```python
from build123d import *
from OCP.BRepFilletAPI import BRepFilletAPI_MakeChamfer

# Parameters (mm, degrees)
SKETCH1_W                 = 5
SKETCH1_H                 = 1.629773482
SKETCH1_H_2               = 1.605700765
BOSS_EXTRUDE21_DEPTH      = 1.5
BOSS_EXTRUDE22_DEPTH      = 0.0001
BOSS_EXTRUDE22_DEPTH_BACK = 5
SKETCH4_W                 = 13.038345926
SKETCH4_H                 = 1.27322458
SKETCH5_W                 = 13.038345926
SKETCH5_H                 = 1.75
BOSS_EXTRUDE23_DEPTH      = 1.5
SKETCH6_W                 = 3.309716912
SKETCH6_H                 = 6.42211522
SKETCH6_W_2               = 3.309716913
BOSS_EXTRUDE24_DEPTH      = 3
SKETCH8_W                 = 3.309716912
SKETCH8_H                 = 1.8
SKETCH8_W_2               = 3.309716913
BOSS_EXTRUDE26_DEPTH      = 1.5
FILLET1_R                 = 1
FILLET2_R                 = 1
CHAMFER1_SIZE             = 3
CHAMFER1_SIZE_2           = 5.412143266


with BuildPart() as part:
    # Sketch1 → Boss-Extrude21 (new body)
    # profile 1 of 3: a face of its own
    with BuildSketch(Plane(origin=(0, 0, 0), x_dir=(1, 0, 0), z_dir=(0, 1, 0))):
        with Locations((9.977336143, 2.209185976)):
            Rectangle(SKETCH1_W, SKETCH1_H)
    # profile 2 of 3: a face of its own
    with BuildSketch(Plane(origin=(0, 0, 0), x_dir=(1, 0, 0), z_dir=(0, 1, 0))):
        Polygon((-7.422672964, -10.702702703), (-20.313450574, -10.702702703), (-20.313450574, -9.652730884), (13.867336143, -9.652730884), (13.867336143, -10.702702703), (0.977336143, -10.702702703), (0.977336143, -11.975927283), (21.477336143, -11.975927283), (21.477336143, 3.024072717), (12.477336143, 3.024072717), (12.477336143, 1.394299235), (7.477336143, 1.394299235), (7.477336143, 3.024072717), (-27.922663857, 3.024072717), (-27.922663857, -11.975927283), (-7.422672964, -11.975927283), align=None)
        with Locations((-16.422663857, 2.186483824)):
            Rectangle(SKETCH1_W, SKETCH1_H_2, mode=Mode.SUBTRACT)
    # profile 3 of 3: a face of its own
    with BuildSketch(Plane(origin=(0, 0, 0), x_dir=(1, 0, 0), z_dir=(0, 1, 0))):
        with Locations((-16.422663857, 2.186483824)):
            Rectangle(SKETCH1_W, SKETCH1_H_2)
    extrude(amount=BOSS_EXTRUDE21_DEPTH)

    # Sketch4 → Boss-Extrude22 (add, two sides: drawn at the far end of the back side and taken through both)
    with BuildSketch(Plane.XZ.offset(-BOSS_EXTRUDE22_DEPTH_BACK)):
        with Locations((-0.903500001, 11.339314993)):
            Rectangle(SKETCH4_W, SKETCH4_H)
    extrude(amount=BOSS_EXTRUDE22_DEPTH + BOSS_EXTRUDE22_DEPTH_BACK)

    # Sketch5 → Boss-Extrude23 (add)
    with BuildSketch(Plane.XY.offset(11.975927283)):
        with Locations((-0.903500001, 4.125)):
            Rectangle(SKETCH5_W, SKETCH5_H)
    extrude(amount=BOSS_EXTRUDE23_DEPTH)

    # Sketch6 → Boss-Extrude24 (add)
    with BuildSketch(Plane(origin=(0, 1.5, 0), x_dir=(1, 0, 0), z_dir=(0, 1, 0))):
        with Locations((14.622477687, -0.186984893)):
            Rectangle(SKETCH6_W, SKETCH6_H)
        with Locations((-21.0678054, -0.186984893)):
            Rectangle(SKETCH6_W_2, SKETCH6_H)
    extrude(amount=BOSS_EXTRUDE24_DEPTH)

    # Sketch8 → Boss-Extrude26 (add)
    with BuildSketch(Plane(origin=(0, 0, -3.024072717), x_dir=(-1, 0, 0), z_dir=(0, 0, -1))):
        with Locations((-14.622477687, 3.6)):
            Rectangle(SKETCH8_W, SKETCH8_H)
        with Locations((21.0678054, 3.6)):
            Rectangle(SKETCH8_W_2, SKETCH8_H)
    extrude(amount=BOSS_EXTRUDE26_DEPTH)

    # Fillet1
    fillet1_edges = [part.edges().sort_by_distance(p)[0] for p in [
        (14.622477687, 4.5, -4.524072717),
        (-21.0678054, 4.5, -4.524072717),
        (-0.903500001, 5, 13.475927283),
    ]]
    fillet(fillet1_edges, radius=FILLET1_R)

    # Fillet2
    fillet2_edges = [part.edges().sort_by_distance(p)[0] for p in [
        (21.477336143, 0.75, 11.975927283),
        (-27.922663857, 0.75, 11.975927283),
        (-27.922663857, 0.75, -3.024072717),
        (21.477336143, 0.75, -3.024072717),
    ]]
    fillet(fillet2_edges, radius=FILLET2_R)

    # Chamfer1
    chamfer1_edges_1 = [part.edges().sort_by_distance(p)[0] for p in [
        (14.622477687, 4.5, 3.398042503),
    ]]
    chamfer1_side_1 = [part.faces().sort_by_distance(p)[0] for p in [
        (14.622477687, 4.44, 3.398042503),
    ]]
    chamfer1_edges_2 = [part.edges().sort_by_distance(p)[0] for p in [
        (-21.0678054, 4.5, 3.398042503),
    ]]
    chamfer1_side_2 = [part.faces().sort_by_distance(p)[0] for p in [
        (-21.0678054, 4.44, 3.398042503),
    ]]
    chamfer1 = BRepFilletAPI_MakeChamfer(part.part.solid().wrapped)
    for e in chamfer1_edges_1:
        chamfer1.Add(CHAMFER1_SIZE - 0.0001, CHAMFER1_SIZE_2 - 0.0001, e.wrapped, chamfer1_side_1[0].wrapped)
    for e in chamfer1_edges_2:
        chamfer1.Add(CHAMFER1_SIZE - 0.0001, CHAMFER1_SIZE_2 - 0.0001, e.wrapped, chamfer1_side_2[0].wrapped)
    add(Compound.cast(chamfer1.Shape()), mode=Mode.REPLACE)  # a hair under: the kernel refuses the full size


solid = part.part
```
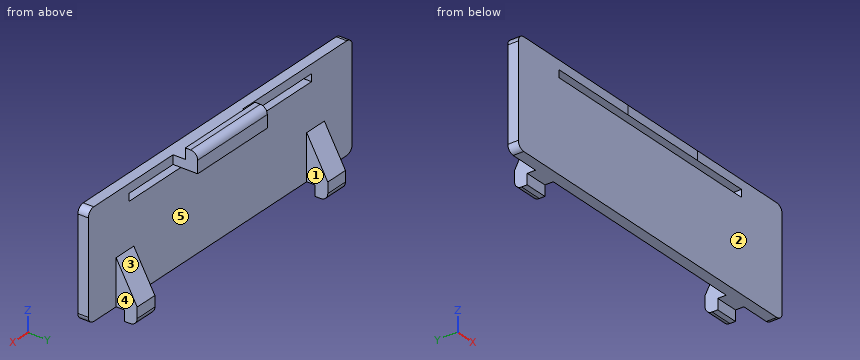
For this review, take the finished solid that the model builds, in its own axes (mm). Face numbers are marked on the shaded views. A direction names the side the tool comes from. Give positions to 0.01 mm unless a question says otherwise; leave off trailing zeros. Write each loop counter-clockwise with the first axis right and the second up, starting at its lowest first coordinate (ties: lowest second). Pieces come first, ordered by that corner, then holes.
Item 1: Take a section at D-D (x = 12.5). Give the boundary of the cut face in (y, z), and give its area (3 significant figures).
Item 2: Machinability: for the marked faces 1 and 2, which of the approach directions +Z, -Z, +X, -X, +Y, -Y give a long, thin tool a straight path to every point of the face, cutting with its end or side? Answer none if there is none.
Item 3: Take a section at A-A (x = -6). Give the boundary of the cut face in (y, z), and give its area (3 significant figures).
Item 4: Insertion check: P1, Ø8, axis at x = 13.5, z = -1, coming from the -Y side; P2, Ø0.5, axis at x = 15, z = -2.5, coming from the +Y side; P3, Ø0.9, axis at y = 3.5, z = -2, coming from the +X side; P4, Ø1.5, axis at x = 14, z = -0.5, coming from the +Y side. Each pin has a flat end and moves straight along its axis. Give the tip position at first contact, or say it passes through.
Item 5: Wall thickness on probe 1 along X at (y, z) = (1.95, 0); probe 2 along Z at (x, y) = (6, 0.45); probe 3 along Y at (x, z) = (1.5, 9.25): over which ranges is each line inside the solid? List them lowest first.
Item 6: The part is to be moulded in two halves that separate along X. For the marked faces 3, 4 and 5, say which applies: +X half, -X half, draft (parallel to the pull), parting line (faces both ways), or undercut.
Item 7: Take a section at C-C (z = 2.75). Give the boundary of the cut face in (x, y), and give its area (3 significant figures).
Established:
1. outline: (0, -3.02) - (1.5, -3.02) - (1.5, 9.65) - (0, 9.65) - close; (0, 10.7) - (1.5, 10.7) - (1.5, 11.98) - (0, 11.98) - close
1. area: 20.9 mm2
2. face 1: +Z, -Z, +Y
2. face 2: +Z, -Z, +X, -X, -Y
3. outline: (0, -3.02) - (1.5, -3.02) - (1.5, 9.65) - (0, 9.65) - close; (0, 10.7) - (5, 10.7) - (5, 12.48) arc R1 ccw to (4, 13.48) - (3.25, 13.48) - (3.25, 11.98) - (0, 11.98) - close
3. area: 27.8 mm2
4. P1: stops at y = 0
4. P2: stops at y = 4.5
4. P3: stops at x = 16.28
4. P4: stops at y = 4.08
5. probe 1: x = -22.72 to -19.41, 12.97 to 16.28
5. probe 2: z = -3.02 to 9.65, 10.7 to 11.98
5. probe 3: y = 0 to 1.5
6. face 3: draft
6. face 4: +X half
6. face 5: undercut
7. outline: (-27.92, 0) - (21.48, 0) - (21.48, 1.5) - (16.28, 1.5) - (16.28, 1.86) - (12.97, 1.86) - (12.97, 1.5) - (-19.41, 1.5) - (-19.41, 1.86) - (-22.72, 1.86) - (-22.72, 1.5) - (-27.92, 1.5) - close
7. area: 76.5 mm2
